from build123d import *

# Parameters (mm, degrees)
SKETCH_1_R               = 9.3
EXTRUDE_1_DEPTH          = 15.5
SKETCH_2_W               = 10.704532534
SKETCH_2_H               = 9.5
EXTRUDE_2_DEPTH          = 2.8
SKETCH_3_R               = 6.45
CUT_EXTRUDE_1_DEPTH      = 10.3
CUT_EXTRUDE_1_DEPTH_BACK = 2
SKETCH_4_R               = 4
CUT_EXTRUDE_2_DEPTH      = 17.7


with BuildPart() as part:
    # Эскиз1 → Бобышка-Вытянуть1 (new body)
    with BuildSketch(Plane.XY):
        Circle(SKETCH_1_R)
    extrude(amount=EXTRUDE_1_DEPTH)

    # Эскиз2 → Бобышка-Вытянуть2 (add)
    with BuildSketch(Plane.XY):
        with Locations((-13.347733733, 0)):
            Rectangle(SKETCH_2_W, SKETCH_2_H)
    extrude(amount=EXTRUDE_2_DEPTH)

    # Эскиз3 → Вырез-Вытянуть1 (cut, two sides)
    with BuildSketch(Plane(origin=(0, 0, 0), x_dir=(0, 0, -1), z_dir=(1, 0, 0))) as cut_extrude_1_sk:
        with Locations((-7.75, 0)):
            Circle(SKETCH_3_R)
    extrude(amount=CUT_EXTRUDE_1_DEPTH, mode=Mode.SUBTRACT)
    extrude(cut_extrude_1_sk.sketch, amount=-CUT_EXTRUDE_1_DEPTH_BACK, mode=Mode.SUBTRACT)

    # Эскиз4 → Вырез-Вытянуть2 (cut, through all)
    with BuildSketch(Plane(origin=(-2, 0, 0), x_dir=(0, 0, -1), z_dir=(1, 0, 0))):
        with Locations((-7.75, 0)):
            Circle(SKETCH_4_R)
    extrude(amount=-CUT_EXTRUDE_2_DEPTH, mode=Mode.SUBTRACT)


solid = part.part
CAD build for the part. Positions are in the model's coordinates, mm. A direction names the side the tool comes from. Give positions to 0.01 mm unless a question says otherwise; leave off trailing zeros. Loops run counter-clockwise (first coordinate to the right, second up) from the corner with the lowest first, then second, coordinate; pieces in that order, holes last. Notation, with made-up numbers: M -21,20.5 L 18,20.5 A29 cw 18,59.5 Z; hole C 10,14 d5. An arc over 180 degrees is marked long. One line per question, with ' | ' between items. Start each with the question number.
1. Saw through at A-A on y = 0. Give the cut face in (x, z).
2. Two-plate mould, pull along Z, no slides. Class faces 1 (the face through (-18.7, 0, 1)), 2 (the face through (-13, 0, 2.8)), 3 (the face through (-2, -3, 11)): pulls with the +Z half, pulls with the -Z half, needs draft (parallel to the pull), parting line crosses it, or undercut.
3. Saw through at D-D on x = -14.5. Give the cut face in (y, z), plus the area to 3 significant figures.
4. 3-axis set-ups, long thin cutter, end or side, ignore diameter. For faces 4 (the face through (3.571, 5.439, 4.283)), 5 (the face through (-13, 4.75, 1)), 6 (the face through (-13, -4.75, 1)), 7 (the face through (0, 0, 15.5)), 8 (the face through (-5.599, 0.176, 11.746)): which of +Z, -Z, +X, -X, +Y, -Y reach the whole face in a straight line?
5. Saw through at C-C on x = 0. Give the cut face in (y, z), plus the area to 3 significant figures.
6. Saw through at B-B on z = 7.75. Give the cut face in (x, y), plus the area to 3 significant figures.
7. Flat gauge pins, fed straight in: pin 1 (2 mm diameter, centred on x = -2.5, z = 9, fed in from -Y); pin 2 (1 mm diameter, centred on y = -2, z = 3.5, fed in from +X); pin 3 (3 mm diameter, centred on x = -11.5, z = 2, fed in from -Y). Where does each tip first touch, or does it go through?
8. Probe L1, parallel to Z at x = 2.5, y = 0; L2, parallel to Z at x = -8, y = 0; L3, parallel to Y at x = -15, z = 1.5. List the from-to ranges inside material, lowest first. Write a range as from..to.
Result sheet:
1) outline: M -18.7,0 L 9.3,0 L 9.3,1.3 L -2,1.3 L -2,3.75 L -9.3,3.75 L -9.3,2.8 L -18.7,2.8 Z; M -9.3,11.75 L -2,11.75 L -2,14.2 L 9.3,14.2 L 9.3,15.5 L -9.3,15.5 Z
2) face 1: needs draft | face 2: pulls with the +Z half | face 3: undercut
3) outline: M -4.75,0 L 4.75,0 L 4.75,2.8 L -4.75,2.8 Z | area: 26.6 mm^2
4) face 4: +X | face 5: +Z, -Z, -X, +Y | face 6: +Z, -Z, -X, -Y | face 7: +Z, +X, -X, +Y, -Y | face 8: +X, -X
5) outline: M -9.3,0 L 9.3,0 L 9.3,15.5 L -9.3,15.5 Z; hole C 0,7.75 d12.9 | area: 158 mm^2
6) outline: M -8.4,-4 A9.3 ccw 6.7,-6.45 L -2,-6.45 L -2,-4 Z; M -8.4,4 L -2,4 L -2,6.45 L 6.7,6.45 A9.3 ccw Z | area: 80.4 mm^2
7) pin 1: stops at y = -9.18 | pin 2: stops at x = -2 | pin 3: stops at y = -4.75
8) L1: z = 0..1.3, 14.2..15.5 | L2: z = 0..3.75, 11.75..15.5 | L3: y = -4.75..4.75
